```python
from build123d import *

# Parameters (mm, degrees)
F1_DEPTH = 2
F2_R     = 1.99999


# Not quite as in the source:
# - a fillet or chamfer is up to 0.001 mm smaller than in the source, because OpenCascade refuses the exact size


with BuildPart() as f1:
    # F0 (on Top) → F1 (new body)
    with BuildSketch(Plane.XY):
        with BuildLine():
            Line((-34.2, -12.075), (22.8, -12.075))
            Line((22.8, -12.075), (22.8, -8.15))
            ThreePointArc((22.8, -8.15), (14.65, 0), (22.8, 8.15))
            Line((22.8, 8.15), (22.8, 12.075))
            Line((22.8, 12.075), (-34.2, 12.075))
            Line((-34.2, 12.075), (-34.2, -12.075))
        make_face()
    extrude(amount=F1_DEPTH)

    # F2 (radius 2 in the source; OpenCascade refuses exactly that, so slightly less here)
    f2_edges = [f1.edges().sort_by_distance(p)[0] for p in [
        (-34.2, -12.075, 1),
        (-34.2, 12.075, 1),
        (-34.2, 0, 2),
    ]]
    fillet(f2_edges, radius=F2_R)


solid = f1.part
```
The listing builds one solid part. Answer for the finished solid, in the listing's coordinates (mm). Give positions to 0.01 mm unless a question says otherwise; leave off trailing zeros. Loops run counter-clockwise (first coordinate to the right, second up) from the corner with the lowest first, then second, coordinate; pieces in that order, holes last. Notation, with made-up numbers: M -20,54.25 L 6,54.25 A23 cw 6,82.25 Z; hole C 75.5,-33.5 d6. An arc over 180 degrees is marked long. One line per item, written item: value.
Q1. Find the intervals of material crossed by line 1 (Y direction, x = 18, z = 1.25) (3 decimals); line 2 (X direction, y = 11, z = 0.9); line 3 (X direction, y = -0.25, z = 0.1), in increasing order. Write a range as from..to.
Working result:
line 1: y = -12.075..-6.587, 6.587..12.075
line 2: x = -33.97..22.8
line 3: x = -34.2..14.65
Q2. A cutting plane is placed at B-B on z = 1.7. Determine the outline of the cut face in (x, y) (3 decimals).
Working result:
outline: M -33.254,-11.775 A2 ccw -32.2,-12.075 L 22.8,-12.075 L 22.8,-8.15 A8.15 cw 22.8,8.15 L 22.8,12.075 L -32.2,12.075 A2 ccw -33.254,11.775 Z
Q3. Determine the mould class of faces 1 (the face through (14.65, -0.18, 0.99)), 2 (the face through (-33.329, 11.726, 0.792)), 3 (the face through (-33.329, -11.726, 0.792)), 4 (the face through (-6, 0, 0)) for opening direction Y: +Y half, -Y half, draft (parallel to the pull), parting line (faces both ways), or undercut.
Working result:
face 1: undercut
face 2: +Y half
face 3: -Y half
face 4: draft
